Could you check a few things on this drawing? It's one solid part, dimensions in mm from its lowest x, y, z. A direction names the side the tool comes from. Coordinates: 2 decimals unless noted, no trailing zeros. Order: outer loops, then holes, each group sorted by start corner. A loop starts at its lowest first (then second) coordinate and runs counter-clockwise, first axis right, second up. Notation, with made-up numbers: M 79,18.25 L 104,18.25 A22 ccw 104,52.25 Z; hole C 60.5,71 d9. An arc over 180 degrees is marked long. Answer as CSV lines item,"result". Start each with the question number.
1. Will these pins go through, and if not, where does the flat tip stop? pin 1 (4 mm diameter, centred on x = 15.5, z = 16, fed in from -Y); pin 2 (3 mm diameter, centred on x = 16, z = 23.5, fed in from +Y); pin 3 (4 mm diameter, centred on x = 26.5, z = 8.5, fed in from -Y).
2. I need wall thicknesses on line 1 along Y through (x, z) = (20, 14); line 2 along X through (y, z) = (20.5, 20); line 3 along Y through (x, z) = (24, 42.5). Which ranges of each line are inside material? Lowest first, please. Write a range as from..to.
3. If we section it at D-D (z = 24): List the corners of the cut face in (x, y) for me, plus the area to 3 significant figures.
4. If we section it at B-B (x = 20): List the corners of the cut face in (y, z) for me.
5. On a 3-axis mill with a long thin cutter (end or side, diameter ignored), from which of +Z, -Z, +X, -X, +Y, -Y can I reach the whole of each face in a straight line? I mean the marked faces 1 and 2. Say none if no direction works.
6. If we mould it in two halves opening along X, with no side actions, what happens to the marked faces 3, 4, 5 and 6? For each: released by +X, released by -X, zero draft, split by the parting line, or undercut.
7. If we section it at A-A (y = 20): List the corners of the cut face in (x, z) for me.
8. If we section it at C-C (z = 10): List the corners of the cut face in (x, y) for me, plus the area to 3 significant figures.
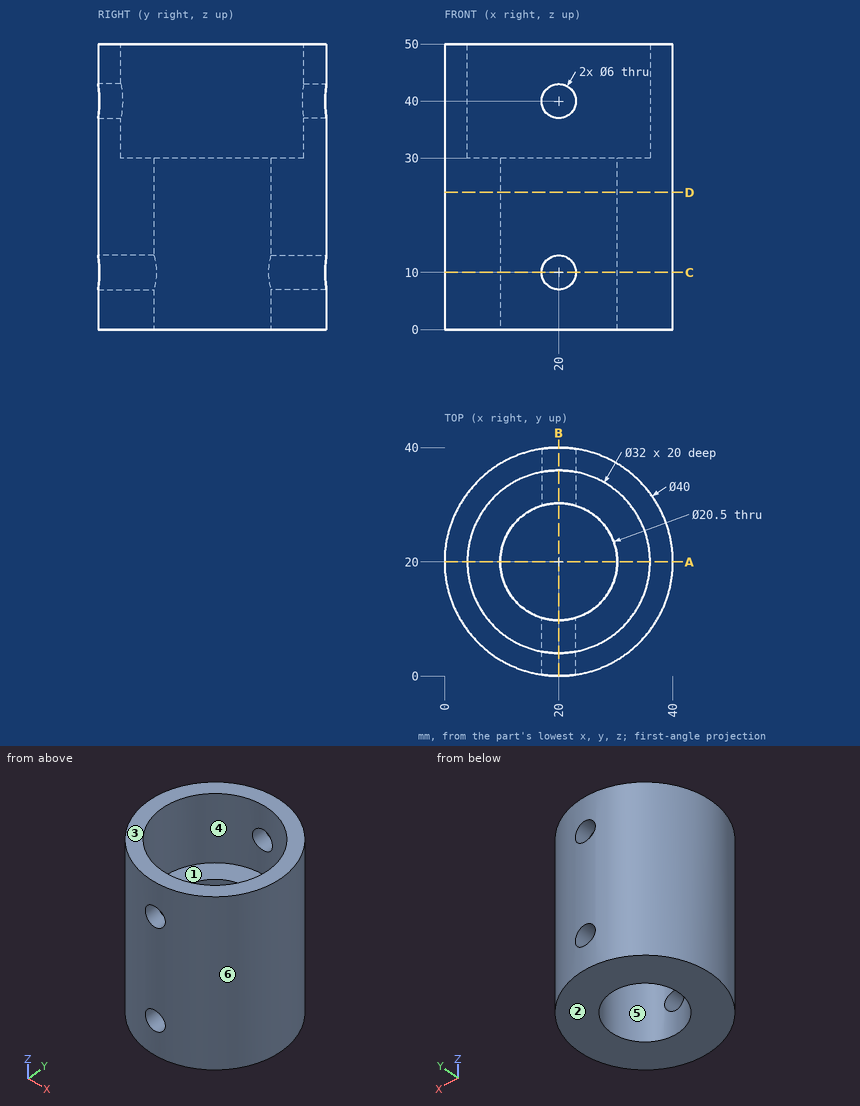
Solved:
1,pin 1,"y = 0.16"
1,pin 2,"y = 39.84"
1,pin 3,"y = 0.51"
2,line 1,"0..9.75, 30.25..40"
2,line 2,"0.01..9.76, 30.24..39.99"
2,line 3,"0.4..4.51, 35.49..39.6"
3,outline,"C 20,20 d40; hole C 20,20 d20.5"
3,area,"927 mm²"
4,outline,"M 0,0 L 9.75,0 L 9.75,7 L 0,7 Z; M 0,13 L 9.75,13 L 9.75,30 L 4,30 L 4,37 L 0,37 Z; M 0,43 L 4,43 L 4,50 L 0,50 Z; M 30.25,0 L 40,0 L 40,7 L 30.25,7 Z; M 30.25,13 L 40,13 L 40,37 L 36,37 L 36,30 L 30.25,30 Z; M 36,43 L 40,43 L 40,50 L 36,50 Z"
5,face 1,"+Z"
5,face 2,"-Z, +X, -X, +Y, -Y"
6,face 3,"zero draft"
6,face 4,"undercut"
6,face 5,"undercut"
6,face 6,"split by the parting line"
7,outline,"M 0,0 L 9.75,0 L 9.75,30 L 4,30 L 4,50 L 0,50 Z; M 30.25,0 L 40,0 L 40,50 L 36,50 L 36,30 L 30.25,30 Z"
8,outline,"M 17,0.23 L 17,10.2 A10.25 cw 17,29.8 L 17,39.77 A20 ccw Z; M 23,0.23 A20 ccw 23,39.77 L 23,29.8 A10.25 cw 23,10.2 Z"
8,area,"809 mm²"
